```python
from build123d import *

# Parameters (mm, degrees)
F0_W     = 7
F0_H     = 5
F0_W_2   = 5
F0_H_2   = 7
F1_DEPTH = 10
F3_DEPTH = 2.5


with BuildPart() as f1:
    # F0 (on Top) → F1 (new body)
    with BuildSketch(Plane.XY):
        Polygon((0, 0), (0, 18.174312), (-7, 18.174312), (-18.174312, 18.174312), (-18.174312, 7), (-18.174312, 0), align=None)
        with Locations((-3.5, 20.674312)):
            Rectangle(F0_W, F0_H)
        Polygon((-7, 23.174312), (0, 23.174312), (0, 25.174312), (-11, 25.174312), (-11, 23.174312), align=None)
        with Locations((-20.674312, 3.5)):
            Rectangle(F0_W_2, F0_H_2)
        Polygon((-25.174312, 0), (-23.174312, 0), (-23.174312, 7), (-23.174312, 12), (-25.174312, 12), align=None)
    extrude(amount=-F1_DEPTH)

    # F2 (on face) → F3 (cut)
    with BuildSketch(Plane.XY):
        with BuildLine():
            Line((0, 0), (0, 15))
            ThreePointArc((0, 15), (-10.606602, 10.606602), (-15, 0))
            Line((-15, 0), (0, 0))
        make_face()
    extrude(amount=-F3_DEPTH, mode=Mode.SUBTRACT)

    # F4: F1 across plane


with BuildPart() as f1_1:
    add(f1.part)
    add(f1.part.mirror(Plane.YZ))

    # F5: F1 across plane


with BuildPart() as f1_2:
    add(f1_1.part)
    add(f1_1.part.mirror(Plane.XZ))


solid = f1_2.part
```
Can you work these out from the model? Positions are in its coordinate system, mm. A direction names the side the tool comes from. Give positions to 0.01 mm unless a question says otherwise; leave off trailing zeros. Loops run counter-clockwise (first coordinate to the right, second up) from the corner with the lowest first, then second, coordinate; pieces in that order, holes last. Notation, with made-up numbers: M 78,15 L 119,15 A22 ccw 119,33 Z; hole C -6,-38.75 d2. An arc over 180 degrees is marked long. Answer in a Markdown table with one row per item.
1. Thinking about a two-plate mould opening in X: for faces 6 (the flat face through (13, 18.174, -5)), 7 (the flat face through (7, -21, -5)), 8 (the flat face through (-23.174, 9, -5)), which applies, released by +X, released by -X, zero draft, split by the parting line, or undercut?
Taken from the geometry:
| item | result |
|---|---|
| face 6 | zero draft |
| face 7 | released by +X |
| face 8 | undercut |
2. For pin 1 Ø4 at (x, z) = (-20.5, -5.5) entering from +Y; pin 2 Ø1.5 at (y, z) = (-18, -4.5) entering from -X; pin 3 Ø2 at (y, z) = (-24, -3) entering from +X, each with a flat end and sliding along its axis, tell me the tip position at first contact or that it passes through.
Taken from the geometry:
| item | result |
|---|---|
| pin 1 | stops at y = 7 |
| pin 2 | stops at x = -18.17 |
| pin 3 | stops at x = 11 |
3. Suppose I cut it at D-D on x = -21.5. Write out the boundary of the cut face in (y, z), plus the area to 3 significant figures.
Taken from the geometry:
| item | result |
|---|---|
| outline | M -7,-10 L 7,-10 L 7,0 L -7,0 Z |
| area | 140 mm² |
4. Which directions (+Z, -Z, +X, -X, +Y, -Y) give clear straight access to the entire face, cutting with the end or side of a thin tool? Please do faces 1 (the flat face through (9, -23.174, -5)), 2 (the flat face through (-13, -18.174, -5)), 3 (the flat face through (-24, 12, -5)), 4 (the flat face through (18.174, 13, -5)), 5 (the flat face through (21, -7, -5)).
Taken from the geometry:
| item | result |
|---|---|
| face 1 | +Z, -Z, +X |
| face 2 | +Z, -Z, -X |
| face 3 | +Z, -Z, -X, +Y |
| face 4 | +Z, -Z, +Y |
| face 5 | +Z, -Z, -Y |
5. Suppose I cut it at A-A on y = 1.5. Write out the boundary of the cut face in (x, z), plus the area to 3 significant figures.
Taken from the geometry:
| item | result |
|---|---|
| outline | M -25.17,-10 L 25.17,-10 L 25.17,0 L 14.92,0 L 14.92,-2.5 L -14.92,-2.5 L -14.92,0 L -25.17,0 Z |
| area | 429 mm² |
6. Suppose I cut it at C-C on y = -16. Write out the boundary of the cut face in (x, z).
Taken from the geometry:
| item | result |
|---|---|
| outline | M -18.17,-10 L 18.17,-10 L 18.17,0 L -18.17,0 Z |
7. If I drill on line 1 along Y through (x, z) = (10, -8.25); line 2 along X through (y, z) = (-15, -4.75), over which ranges is the centre line in solid material (lowest first)?
Taken from the geometry:
| item | result |
|---|---|
| line 1 | y = -25.17 to -23.17, -18.17 to 18.17, 23.17 to 25.17 |
| line 2 | x = -18.17 to 18.17 |
8. Suppose I cut it at B-B on x = 12. Write out the boundary of the cut face in (y, z).
Taken from the geometry:
| item | result |
|---|---|
| outline | M -18.17,-10 L 18.17,-10 L 18.17,0 L 9,0 L 9,-2.5 L -9,-2.5 L -9,0 L -18.17,0 Z |
